```python
from build123d import *

# Parameters (mm, degrees)
F0_R     = 6.35
F1_DEPTH = 3.175
F2_R     = 9.525
F2_R_2   = 6.35
F3_DEPTH = 2.54
F4_R     = 4.445
F5_DEPTH = 2.54


with BuildPart() as f1:
    # F0 (on Front) → F1 (new body)
    with BuildSketch(Plane.XZ):
        Circle(F0_R)
    extrude(amount=F1_DEPTH)

    # F2 (on face) → F3 (join)
    with BuildSketch(Plane.XZ.offset(3.175)):
        Circle(F2_R)
        Circle(F2_R_2, mode=Mode.SUBTRACT)
        Circle(F2_R_2)
    extrude(amount=F3_DEPTH)

    # F4 (on face) → F5 (cut)
    with BuildSketch(Plane(origin=(0, 0, 0), x_dir=(-1, 0, 0), z_dir=(0, 1, 0))):
        Circle(F4_R)
    extrude(amount=-F5_DEPTH, mode=Mode.SUBTRACT)


solid = f1.part
```
Read the model definition and answer for the solid it produces. Units are mm, in the model's axes. A direction names the side the tool comes from. Round coordinates to 2 decimals unless told otherwise and drop trailing zeros. Write each loop counter-clockwise with the first axis right and the second up, starting at its lowest first coordinate (ties: lowest second). Pieces come first, ordered by that corner, then holes. Notation, with made-up numbers: (4, -14) - (42, -14) arc R28 ccw to (42, 13) - close; hole circle Ø4 at (12.5, -3). An arc over 180 degrees is marked (long way). Use CSV: the item, a comma, the result in double quotes.
Q1. Find section C-C, the plane y = -0.95. Write down the section's boundary in (x, z) (3 decimals), then the cut area to 3 significant figures.
Values:
outline,"circle Ø12.7 at (0, 0); hole circle Ø8.89 at (0, 0)"
area,"64.6 mm²"
Q2. Each of these flat-tipped pins is pushed along its axis until it touches: pin 1 Ø1.5 at (y, z) = (-5, 2) entering from +X; pin 2 Ø4.5 at (x, z) = (-0.5, -2) entering from +Y; pin 3 Ø1 at (y, z) = (-4, 7) entering from +X. Where does it stop, or does it pass through?
Values:
pin 1,"stops at x = 9.44"
pin 2,"stops at y = -2.54"
pin 3,"stops at x = 6.96"
Q3. Find section B-B, the plane z = -3.5. Write down the section's boundary in (x, y) (3 decimals), then the cut area to 3 significant figures.
Values:
outline,"(-8.859, -5.715) - (8.859, -5.715) - (8.859, -3.175) - (5.298, -3.175) - (5.298, 0) - (2.74, 0) - (2.74, -2.54) - (-2.74, -2.54) - (-2.74, 0) - (-5.298, 0) - (-5.298, -3.175) - (-8.859, -3.175) - close"
area,"64.7 mm²"
Q4. Straight lines are drawn through the part: line 1 along Z through (x, y) = (0, -1.65) (3 decimals); line 2 along Y through (x, z) = (6.5, 0.25) (3 decimals); line 3 along Z through (x, y) = (-1.75, -2.45). For each, find the intervals that lie inside material, in ascending order.
Values:
line 1,"z = -6.35 to -4.445, 4.445 to 6.35"
line 2,"y = -5.715 to -3.175"
line 3,"z = -6.1 to -4.09, 4.09 to 6.1"
Q5. Find section D-D, the plane y = -3.4. Write down the section's boundary in (x, z) (3 decimals).
Values:
outline,"circle Ø19.05 at (0, 0)"
Q6. Determine the mould class of faces 1 (the cylindrical face through (-7.559, -4.427, -5.796)), 2 (the flat face through (0, -2.54, 0)), 3 (the cylindrical face through (0.96, -1.25, -4.34)), 4 (the flat face through (0, -5.715, 0)) for opening direction Z: +Z half, -Z half, draft (parallel to the pull), parting line (faces both ways), or undercut.
Values:
face 1,"parting line"
face 2,"undercut"
face 3,"undercut"
face 4,"draft"
Q7. Find section A-A, the plane x = 0. Write down the section's boundary in (y, z) (3 decimals), then the cut area to 3 significant figures.
Values:
outline,"(-5.715, -9.525) - (-3.175, -9.525) - (-3.175, -6.35) - (0, -6.35) - (0, -4.445) - (-2.54, -4.445) - (-2.54, 4.445) - (0, 4.445) - (0, 6.35) - (-3.175, 6.35) - (-3.175, 9.525) - (-5.715, 9.525) - close"
area,"66.1 mm²"
Q8. A tool of negligible diameter and unlimited length cuts with its end or side. For faces 5 (the flat face through (2, -3.175, -6.2)), 6 (the flat face through (3, 0, -4)), from which of +Z, -Z, +X, -X, +Y, -Y can it reach the whole face along a straight path? Write none if from no direction.
Values:
face 5,"+Y"
face 6,"+Z, -Z, +X, -X, +Y"
